Here's the drawing with two shaded views (mm, measured from the low corner). I have some questions. A direction names the side the tool comes from. Coordinates: 2 decimals unless noted, no trailing zeros. Loops run counter-clockwise (first coordinate to the right, second up) from the corner with the lowest first, then second, coordinate; pieces in that order, holes last.
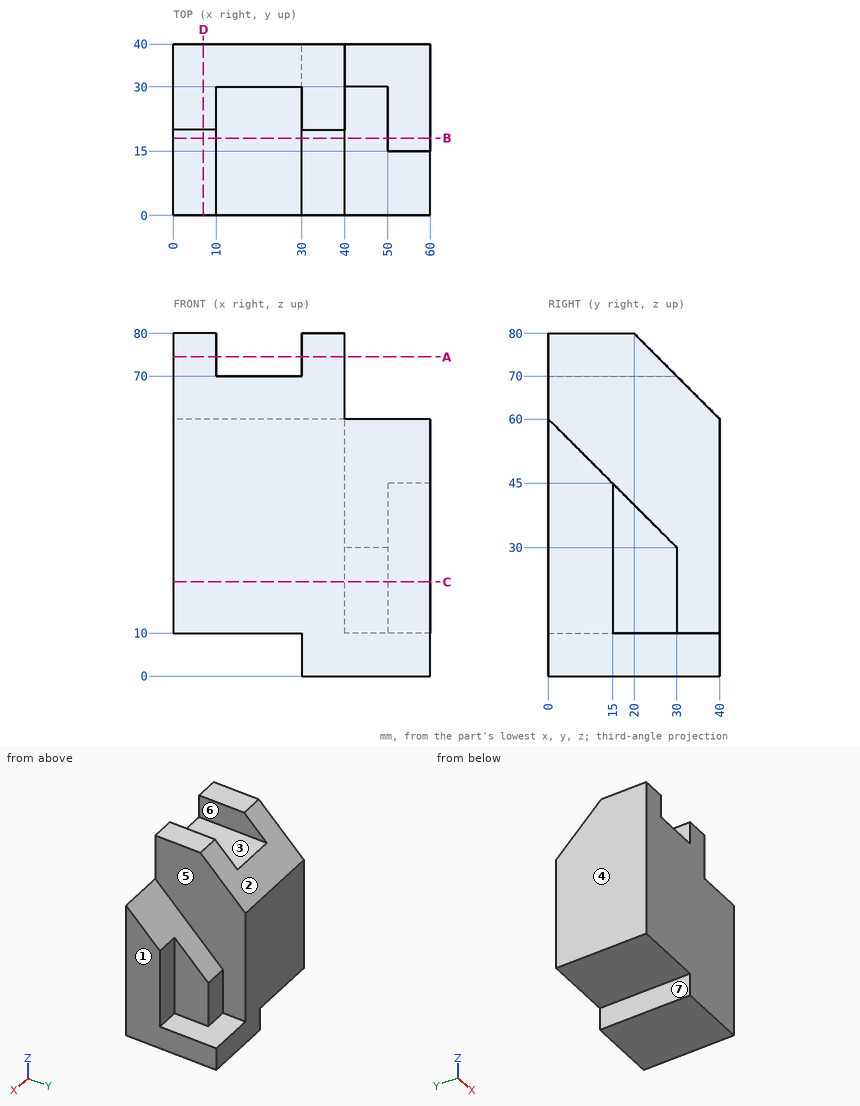
(1) If I drill on probe 1 along X at (y, z) = (17.5, 76); probe 2 along Z at (x, y) = (16, 24.5); probe 3 along Y at (x, z) = (41, 24), over which ranges is the centre line in solid material (lowest first)?
Check values:
probe 1: x = 0 to 10, 30 to 40
probe 2: z = 10 to 70
probe 3: y = 0 to 30
(2) I want a section at D-D on x = 7. Write out the boundary of the cut face in (y, z), then the cut area to 3 significant figures.
Check values:
outline: (0, 10) - (40, 10) - (40, 60) - (20, 80) - (0, 80) - close
area: 2,600 mm2
(3) If we mould it in two halves opening along X, with no side actions, what happens to the marked faces 1, 2, 3 and 4? For each: released by +X, released by -X, zero draft, split by the parting line, or undercut.
Check values:
face 1: released by +X
face 2: zero draft
face 3: undercut
face 4: released by -X
(4) I want a section at B-B on y = 18. Write out the boundary of the cut face in (x, z), then the cut area to 3 significant figures.
Check values:
outline: (0, 10) - (30, 10) - (30, 0) - (60, 0) - (60, 10) - (50, 10) - (50, 42) - (40, 42) - (40, 80) - (30, 80) - (30, 70) - (10, 70) - (10, 80) - (0, 80) - close
area: 3,220 mm2
(5) I want a section at C-C on z = 22. Write out the boundary of the cut face in (x, y), then the cut area to 3 significant figures.
Check values:
outline: (0, 0) - (60, 0) - (60, 15) - (50, 15) - (50, 30) - (40, 30) - (40, 40) - (0, 40) - close
area: 2,050 mm2
(6) Which directions (+Z, -Z, +X, -X, +Y, -Y) give clear straight access to the entire face, cutting with the end or side of a thin tool? Please do the marked faces 5, 6 and 7.
Check values:
face 5: +Z, +X, +Y
face 6: +Z, +Y, -Y
face 7: -Z, -X, +Y, -Y
(7) I want a section at A-A on z = 74.5. Write out the boundary of the cut face in (x, y).
Check values:
outline: (0, 0) - (10, 0) - (10, 25.5) - (0, 25.5) - close; (30, 0) - (40, 0) - (40, 25.5) - (30, 25.5) - close
(8) I'm going to push flat-ended pins straight in: pin 1 (5 mm diameter, centred on y = 11.5, z = 76.5, fed in from +X); pin 2 (3 mm diameter, centred on y = 13, z = 4.5, fed in from -X); pin 3 (3 mm diameter, centred on x = 8.5, y = 9, fed in from -Z); pin 4 (22 mm diameter, centred on x = 20, y = 10.5, fed in from +Z). Where does each tip first touch, or does it pass through?
Check values:
pin 1: stops at x = 40
pin 2: stops at x = 30
pin 3: stops at z = 10
pin 4: stops at z = 80
